Verification items for the finished model (mm, model axes). Give positions to 0.01 mm unless a question says otherwise; leave off trailing zeros. Order: outer loops, then holes, each group sorted by start corner. A loop starts at its lowest first (then second) coordinate and runs counter-clockwise, first axis right, second up.
(1) Sectioned sample at A-A on x = -145. Record the cut outline in (y, z).
(2) Gauge pin test, flat ends, axial feed: pin 1 (1.2 mm diameter, centred on x = -35, y = -2, fed in from -Z); pin 2 (1.5 mm diameter, centred on x = -221, y = -5, fed in from -Z); pin 3 (1.5 mm diameter, centred on x = -4.53, z = 0, fed in from +Y); pin 4 (1.2 mm diameter, centred on x = -27.5, y = -2, fed in from +Z). Record the tip position at first contact, or that the pin passes through.
(3) Sectioned sample at B-B on y = 3.75. Record the cut outline in (x, z), plus the area to 3 significant figures.
(4) Scan lines: L1, parallel to X at y = -3.5, z = 0; L2, parallel to X at y = 4.25, z = -3.75; L3, parallel to Z at x = -199, y = -0.25. Record each from-to range of solid material in increasing order.
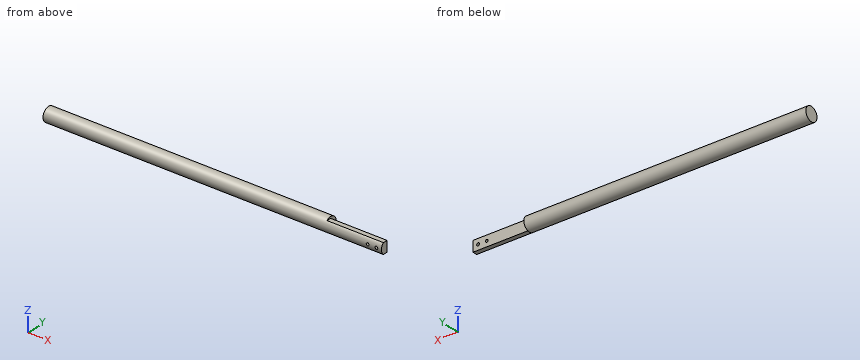
Autodesk Inventor part; units mm, degrees
ref_plane "YZ Plane" through (0, 0, 0) normal (1, 0, 0) x (0, 1, 0)
ref_plane "XZ Plane" through (0, 0, 0) normal (0, 1, 0) x (-1, 0, 0)
ref_plane "XY Plane" through (0, 0, 0) normal (0, 0, 1) x (1, 0, 0)
sketch "Sketch1" plane through (0, 0, 0) normal (1, 0, 0) x (0, 1, 0)
  circle A0 centre (0, 0) radius 6.35
  dimension "d61" = 12.7
extrude "Extrusion1" add sketch "Sketch1" against normal blind 304.8
sketch "Sketch2" plane through (0, 0, 0) normal (1, 0, 0) x (0, 0, -1)
  arc A0 (6.35, 0) -> (-6.35, 0) centre (0, 0) ccw
  circle A1 centre (0, 0) radius 6.35
  line L0 (-6.35, 0) -> (6.35, 0)
extrude "Extrusion2" cut sketch "Sketch2" against normal blind 50.8 contours L0 A0
sketch "Sketch3" plane through (0, 0, 6.35) normal (0, 1, 0) x (1, 0, 0)
  circle A0 centre (-12.468, 6.35) radius 1.5875
  circle A1 centre (-4.5305, 6.35) radius 1.5875
  line L0 (0, 6.35) -> (-2.943, 6.35)
  line L1 (0, 12.7) -> (0, 0)
  line L2 (-2.943, 6.35) -> (-12.468, 6.35) construction
  dimension "d50" = 3.175
  dimension "d48" = 7.9375
  dimension "d49" = 3.175
  dimension "d60" = 2.943
sketch "Sketch5" plane through (0, 0, 6.35) normal (0, 1, 0) x (1, 0, 0)
  line L0 (0, 6.35) -> (0, 11.176)
  line L1 (0, 12.7) -> (0, 0)
  line L2 (0, 11.176) -> (-50.8, 11.176)
  line L3 (-50.8, 12.7) -> (-50.8, 0)
  line L4 (0, 6.35) -> (0, 1.524)
  line L5 (0, 1.524) -> (-50.8, 1.524)
  line L6 (-50.8, 1.524) -> (-50.8, -4.826)
  line L7 (-50.8, -4.826) -> (10.9985, -4.826)
  line L8 (10.9985, -4.826) -> (0, 1.524)
  line L9 (-50.8, 11.176) -> (-50.8, 17.526)
  line L10 (-50.8, 17.526) -> (10.9985, 17.526)
  line L11 (0, 11.176) -> (10.9985, 17.526)
  line L12 (-50.8, 12.7) -> (0, 12.7)
  dimension "d20" = 4.826
  dimension "d21" = 4.826
  dimension "d62" = 4.826
extrude "Extrusion3" cut sketch "Sketch5" against normal blind 25.4 contours L2 L3 L12 L1 | L1 L12 L9 L10 L11 | L8 L7 L6 L3 L5
hole "Hole3" at (-12.468, 0, 0) at (-4.5305, 0, 0) direction (0, -1, 0) diameter 2.4867 end through all
equation "\"d62\" = d20"
properties part number "rat_headbarStraight" material "Stainless Steel"
Ans:
1. outline: circle Ø12.7 at (0, 0)
2. pin 1: stops at z = -4.83
2. pin 2: stops at z = -4.72
2. pin 3: passes through
2. pin 4: stops at z = 4.83
3. outline: (-304.8, -5.12) - (-50.8, -5.12) - (-50.8, 5.12) - (-304.8, 5.12) - close
3. area: 2,600 mm2
4. L1: x = -304.8 to -13.71, -11.22 to -5.77, -3.29 to 0
4. L2: x = -304.8 to -50.8
4. L3: z = -6.35 to 6.35
